Design review of the part built by this model. Coordinates are the model's own, in mm. Coordinates: 2 decimals unless noted, no trailing zeros. Write each loop counter-clockwise with the first axis right and the second up, starting at its lowest first coordinate (ties: lowest second). Pieces come first, ordered by that corner, then holes. Notation, with made-up numbers: (16, 40) -> (62, 40) arc R22 cw to (62, 58) -> close; hole circle Ø9 at (16, 20). An arc over 180 degrees is marked (long way). Return JSON: item names as keys, results as strings. Group by question number.
from build123d import *

# Parameters (mm, degrees)
F0_W     = 114.3
F0_H     = 19.05
F1_DEPTH = 38.1
F2_R     = 19.04999
F3_R     = 9.525
F4_DEPTH = 38.1


# Not quite as in the source:
# - a fillet or chamfer is up to 0.001 mm smaller than in the source, because OpenCascade refuses the exact size


with BuildPart() as f1:
    # F0 (on Front) → F1 (new body)
    with BuildSketch(Plane.XZ):
        with Locations((-4.4788396761, 9.525)):
            Rectangle(F0_W, F0_H)
    extrude(amount=F1_DEPTH)

    # F2 (radius 19.05 in the source; OpenCascade refuses exactly that, so slightly less here)
    f2_edges = [f1.edges().sort_by_distance(p)[0] for p in [
        (52.67116, -38.1, 9.525),
        (52.67116, 0, 9.525),
    ]]
    fillet(f2_edges, radius=F2_R)

    # F3 (on face) → F4 (cut)
    with BuildSketch(Plane.XY.offset(19.05)):
        with Locations((-42.5788396761, -19.05)):
            Circle(F3_R)
        with Locations((20.9211603239, -20.5131974071)):
            Circle(F3_R)
    extrude(amount=-F4_DEPTH, mode=Mode.SUBTRACT)


solid = f1.part
Q1. The part is to be moulded in two halves that separate along Y. For faces 1 (the cylindrical face through (47.24, -5.73, 9.66)), 2 (the flat face through (-5, -19, 19.05)), 3 (the cylindrical face through (25.32, -28.96, 9.66)), say which applies: +Y half, -Y half, draft (parallel to the pull), parting line (faces both ways), or undercut.
Q2. We need section D-D on x = 22.5. Write out the cut boundary in (y, z), plus the area to 3 significant figures.
Q3. We need section C-C on z = 6.5. State how many separate pieces and enclosed holes the cut face has, plus the area to 3 significant figures.
Q4. We need section A-A on x = -42. Write out the cut boundary in (y, z), plus the area to 3 significant figures.
Q5. For P1, Ø6, axis at y = -10.5, z = 3, coming from the +X side; P2, Ø1, axis at y = -9.5, z = 15, coming from the +X side, all flat-tipped, find the tip position at first contact; note any pin that passes through.
Q6. Wall thickness on L1, parallel to X at y = -16, z = 12; L2, parallel to X at y = -21.5, z = 8.5; L3, parallel to Y at x = 29, z = 5.25: over which ranges is each line inside the solid? List them lowest first.
Q7. We need section B-B on y = -15. Write out the cut boundary in (x, z).
Findings below:
{
 "1": {"face 1": "+Y half", "face 2": "draft", "face 3": "undercut"},
 "2": {"outline": "(-38.1, 0) -> (-29.91, 0) -> (-29.91, 19.05) -> (-38.1, 19.05) -> close; (-11.12, 0) -> (0, 0) -> (0, 19.05) -> (-11.12, 19.05) -> close", "area": "368 mm^2"},
 "3": {"separate pieces": "1", "enclosed holes": "2", "area": "3,630 mm^2"},
 "4": {"outline": "(-38.1, 0) -> (-28.56, 0) -> (-28.56, 19.05) -> (-38.1, 19.05) -> close; (-9.54, 0) -> (0, 0) -> (0, 19.05) -> (-9.54, 19.05) -> close", "area": "364 mm^2"},
 "5": {"P1": "stops at x = 51.84", "P2": "stops at x = 50.38"},
 "6": {"L1": "x = -61.63 to -51.6, -33.56 to 12.53, 29.31 to 52.43", "L2": "x = -61.63 to -51.78, -33.37 to 11.45, 30.39 to 52.51", "L3": "y = -38.1 to -25.56, -15.47 to 0"},
 "7": {"outline": "(-61.63, 0) -> (-51.2, 0) -> (-51.2, 19.05) -> (-61.63, 19.05) -> close; (-33.96, 0) -> (13.15, 0) -> (13.15, 19.05) -> (-33.96, 19.05) -> close; (28.69, 0) -> (52.24, 0) -> (52.24, 19.05) -> (28.69, 19.05) -> close"}
}
